from build123d import *

# Parameters (mm, degrees)
SKETCH1_W           = 58.28
SKETCH1_H           = 99
SKETCH1_W_2         = 5.14
SKETCH1_H_2         = 25.4
BOSS_EXTRUDE1_DEPTH = 2
SKETCH2_W           = 4
SKETCH2_H           = 40
BOSS_EXTRUDE2_DEPTH = 20
CUT_EXTRUDE1_REACH  = 107.741
SKETCH3_R           = 2.55
CHAMFER1_SIZE       = 2
CUT_EXTRUDE2_REACH  = 107.741
CUT_EXTRUDE3_DEPTH  = 2


with BuildPart() as part:
    # Sketch1 → Boss-Extrude1 (new body)
    with BuildSketch(Plane(origin=(0, 0, 0), x_dir=(1, 0, 0), z_dir=(0, 1, 0))):
        with Locations((24.14, 44.5)):
            Rectangle(SKETCH1_W, SKETCH1_H)
        with Locations((2.57, 76.3)):
            Rectangle(SKETCH1_W_2, SKETCH1_H_2, mode=Mode.SUBTRACT)
        with Locations((45.71, 76.3)):
            Rectangle(SKETCH1_W_2, SKETCH1_H_2, mode=Mode.SUBTRACT)
        with Locations((2.57, 12.7)):
            Rectangle(SKETCH1_W_2, SKETCH1_H_2, mode=Mode.SUBTRACT)
        with Locations((45.71, 12.7)):
            Rectangle(SKETCH1_W_2, SKETCH1_H_2, mode=Mode.SUBTRACT)
    extrude(amount=BOSS_EXTRUDE1_DEPTH)

    # Sketch2 → Boss-Extrude2 (add)
    with BuildSketch(Plane(origin=(0, 2, 0), x_dir=(1, 0, 0), z_dir=(0, 1, 0))):
        with Locations((12.14, 44.5)):
            Rectangle(SKETCH2_W, SKETCH2_H)
        with Locations((36.14, 44.5)):
            Rectangle(SKETCH2_W, SKETCH2_H)
    extrude(amount=BOSS_EXTRUDE2_DEPTH)

    # Cut-Extrude1: up to this face of the body (flat: up to its plane)
    cut_extrude1_end = Plane(part.part.faces().sort_by_distance((10.14, 12, -44.5))[0])
    # Sketch3 → Cut-Extrude1 (cut, up to the picked face)
    with BuildSketch(Plane(origin=(38.14, 0, 0), x_dir=(0, 0, -1), z_dir=(1, 0, 0)), mode=Mode.PRIVATE) as cut_extrude1_sk1:
        with Locations((39.5, 12)):
            Circle(SKETCH3_R)
    cut_extrude1_tool1 = split(extrude(cut_extrude1_sk1.sketch, amount=-CUT_EXTRUDE1_REACH, mode=Mode.PRIVATE), bisect_by=cut_extrude1_end, keep=Keep.BOTH, mode=Mode.PRIVATE)
    # Sketch3 → Cut-Extrude1 (cut, up to the picked face)
    with BuildSketch(Plane(origin=(38.14, 0, 0), x_dir=(0, 0, -1), z_dir=(1, 0, 0)), mode=Mode.PRIVATE) as cut_extrude1_sk2:
        with Locations((49.5, 12)):
            Circle(SKETCH3_R)
    cut_extrude1_tool2 = split(extrude(cut_extrude1_sk2.sketch, amount=-CUT_EXTRUDE1_REACH, mode=Mode.PRIVATE), bisect_by=cut_extrude1_end, keep=Keep.BOTH, mode=Mode.PRIVATE)
    add(cut_extrude1_tool1.solids().sort_by(Axis((38.14, 12, -39.5), (-1, 0, 0)))[0], mode=Mode.SUBTRACT)
    add(cut_extrude1_tool2.solids().sort_by(Axis((38.14, 12, -49.5), (-1, 0, 0)))[0], mode=Mode.SUBTRACT)

    # Chamfer1
    chamfer1_edges = [part.edges().sort_by_distance(p)[0] for p in [
        (12.14, 2, -64.5),
        (10.14, 2, -44.5),
        (12.14, 2, -24.5),
        (36.14, 2, -24.5),
        (38.14, 2, -44.5),
        (36.14, 2, -64.5),
    ]]
    chamfer(chamfer1_edges, length=CHAMFER1_SIZE)

    # Cut-Extrude2: up to this face of the body (flat: up to its plane)
    cut_extrude2_end = Plane(part.part.faces().sort_by_distance((38.14, 13.060158725, -44.5))[0])
    # Sketch4 → Cut-Extrude2 (cut, up to the picked face)
    with BuildSketch(Plane.ZY.offset(-10.14), mode=Mode.PRIVATE) as cut_extrude2_sk1:
        Polygon((-55.5, 22), (-64.5, 13), (-64.5, 22), align=None)
    cut_extrude2_tool1 = split(extrude(cut_extrude2_sk1.sketch, amount=-CUT_EXTRUDE2_REACH, mode=Mode.PRIVATE), bisect_by=cut_extrude2_end, keep=Keep.BOTH, mode=Mode.PRIVATE)
    # Sketch4 → Cut-Extrude2 (cut, up to the picked face)
    with BuildSketch(Plane.ZY.offset(-10.14), mode=Mode.PRIVATE) as cut_extrude2_sk2:
        Polygon((-33.5, 22), (-24.5, 13), (-24.5, 22), align=None)
    cut_extrude2_tool2 = split(extrude(cut_extrude2_sk2.sketch, amount=-CUT_EXTRUDE2_REACH, mode=Mode.PRIVATE), bisect_by=cut_extrude2_end, keep=Keep.BOTH, mode=Mode.PRIVATE)
    add(cut_extrude2_tool1.solids().sort_by(Axis((10.14, 19, -61.5), (1, 0, 0)))[0], mode=Mode.SUBTRACT)
    add(cut_extrude2_tool2.solids().sort_by(Axis((10.14, 19, -27.5), (1, 0, 0)))[0], mode=Mode.SUBTRACT)

    # Sketch5 → Cut-Extrude3 (cut)
    with BuildSketch(Plane(origin=(0, 2, 0), x_dir=(1, 0, 0), z_dir=(0, 1, 0))):
        Polygon((34.14, 22.5), (34.14, 66.5), (34.14, 71.5), (40.14, 71.5), (40.14, 89), (8.14, 89), (8.14, 71.5), (14.14, 71.5), (14.14, 66.5), (14.14, 22.5), (14.14, 17.5), (8.14, 17.5), (8.14, 0), (40.14, 0), (40.14, 17.5), (34.14, 17.5), align=None)
    extrude(amount=-CUT_EXTRUDE3_DEPTH, mode=Mode.SUBTRACT)


solid = part.part
Geometry: final body of the model. Coordinates: model frame, mm. A direction names the side the tool comes from. Give positions to 0.01 mm unless a question says otherwise; leave off trailing zeros. Order: outer loops, then holes, each group sorted by start corner. A loop starts at its lowest first (then second) coordinate and runs counter-clockwise, first axis right, second up. Notation, with made-up numbers: (-2, 53) -> (32, 53) arc R28 ccw to (32, 73) -> close; hole circle Ø7 at (13, 23.25). An arc over 180 degrees is marked (long way). Put each result on its own line as item: value.
Q1. Reachability of faces 1 (the face through (36, 8, -64.5)), 2 (the face through (36, 8, -24.5)), 3 (the face through (24, 1, -94)), 4 (the face through (48.28, 1, -76)) from +Z, -Z, +X, -X, +Y, -Y: full face, straight path, thin tool, end or side. Return the list, or none.
Here are the results:
face 1: -Z, +X, -X, +Y
face 2: +Z, +X, -X, +Y
face 3: -Z, +X, -X, +Y, -Y
face 4: +Y, -Y
Q2. Section C-C, the plane z = -11. Return loops of the section in (x, y), then the cut area to 3 significant figures.
Here are the results:
outline: (-5, 0) -> (0, 0) -> (0, 2) -> (-5, 2) -> close; (5.14, 0) -> (8.14, 0) -> (8.14, 2) -> (5.14, 2) -> close; (40.14, 0) -> (43.14, 0) -> (43.14, 2) -> (40.14, 2) -> close; (48.28, 0) -> (53.28, 0) -> (53.28, 2) -> (48.28, 2) -> close
area: 32.0 mm^2
Q3. Draft query along Y for faces 5 (the face through (11, 1, -17.5)), 6 (the face through (36.1, 17.6, -29.1)), 7 (the face through (12.168, 12.112, -36.952)), 8 (the face through (36.168, 12.112, -46.952)). Return one class per face: released by +Y, released by -Y, zero draft, split by the parting line, or undercut.
Here are the results:
face 5: zero draft
face 6: released by +Y
face 7: undercut
face 8: undercut
Q4. Material intervals for L1, parallel to Y at x = 11.05, z = -49.5; L2, parallel to X at y = 12.75, z = -27; L3, parallel to Y at x = 6.5, z = -4, sorted ascending.
Here are the results:
L1: y = 0 to 9.45, 14.55 to 22
L2: x = 10.14 to 14.14, 34.14 to 38.14
L3: y = 0 to 2
Q5. Section B-B, the plane y = 12. Return loops of the section in (x, z).
Here are the results:
outline: (10.14, -64.5) -> (14.14, -64.5) -> (14.14, -52.05) -> (10.14, -52.05) -> close; (10.14, -46.95) -> (14.14, -46.95) -> (14.14, -42.05) -> (10.14, -42.05) -> close; (10.14, -36.95) -> (14.14, -36.95) -> (14.14, -24.5) -> (10.14, -24.5) -> close; (34.14, -64.5) -> (38.14, -64.5) -> (38.14, -52.05) -> (34.14, -52.05) -> close; (34.14, -46.95) -> (38.14, -46.95) -> (38.14, -42.05) -> (34.14, -42.05) -> close; (34.14, -36.95) -> (38.14, -36.95) -> (38.14, -24.5) -> (34.14, -24.5) -> close
Q6. Section D-D, the plane x = 24.5. Return loops of the section in (y, z), then the cut area to 3 significant figures.
Here are the results:
outline: (0, -94) -> (2, -94) -> (2, -89) -> (0, -89) -> close; (0, 0) -> (2, 0) -> (2, 5) -> (0, 5) -> close
area: 20.0 mm^2
Q7. Pin query (flat end, axial travel): pin 1 (10 mm diameter, centred on x = 15.5, y = 17, fed in from -Z); pin 2 (12 mm diameter, centred on x = 15, y = 15.5, fed in from +Z); pin 3 (5.5 mm diameter, centred on y = 10, z = -40.5, fed in from -X). Return the tip coordinate at first contact, or that it passes through.
Here are the results:
pin 1: stops at z = -64.5
pin 2: stops at z = -24.5
pin 3: stops at x = 10.14
Q8. Section A-A, the plane z = -61. Return loops of the section in (x, y), then the cut area to 3 significant figures.
Here are the results:
outline: (-5, 0) -> (14.14, 0) -> (14.14, 16.5) -> (10.14, 16.5) -> (10.14, 4) -> (8.14, 2) -> (-5, 2) -> close; (34.14, 0) -> (53.28, 0) -> (53.28, 2) -> (40.14, 2) -> (38.14, 4) -> (38.14, 16.5) -> (34.14, 16.5) -> close
area: 197 mm^2
